Design review of the part built by this model. Coordinates are the model's own, in mm. A direction names the side the tool comes from. Coordinates: 2 decimals unless noted, no trailing zeros. Write each loop counter-clockwise with the first axis right and the second up, starting at its lowest first coordinate (ties: lowest second). Pieces come first, ordered by that corner, then holes. Notation, with made-up numbers: (39.25, 51.25) -> (62.25, 51.25) arc R22 ccw to (62.25, 73.25) -> close; hole circle Ø8 at (-38.5, 70.25). An arc over 180 degrees is marked (long way). One line per question, with ' | ' between items. Start each with the question number.
Q1. Add section C-C on y = 0. State the section outline as (x, z) points, and give its area (3 significant figures).
Q2. For P1, Ø16, axis at x = 17, z = 609, coming from the -Y side; P2, Ø10, axis at x = 46.5, z = 456.5, coming from the +Y side; P3, Ø6, axis at x = 11, y = -98, coming from the -Z side; P4, Ø24, axis at x = 0, z = 730, coming from the +Y side, all flat-tipped, find the tip position at first contact; note any pin that passes through.
Q3. Wall thickness on probe 1 along Z at (x, y) = (0, 104); probe 2 along Y at (x, z) = (-16.5, 681.5); probe 3 along Z at (x, y) = (44, 4): over which ranges is each line inside the solid? List them lowest first.
Q4. For faces 1 (the flat face through (-35, -105, 629)), 2 (the flat face through (35, -105, 629)), 3 (the flat face through (0, 110, 555)), 4 (the flat face through (0, 90, 610)), list the 3-axis set-ups (+Z, -Z, +X, -X, +Y, -Y) from which the entire face can be reached by the end or side of a thin tool; tool diameter is ignored.
Q5. Add section B-B on x = 0. Give the number of separate pieces and of enclosed holes in the cut face, and give its area (3 significant figures).
Q6. Add section A-A on z = 730. State the section outline as (x, y) points, and give its area (3 significant figures).
Q7. Draft analysis for pull direction Y (two halves, no side actions). For faces 5 (the flat face through (0, 120, 692)), 6 (the flat face through (0, 100, 500)), 7 (the flat face through (0, -100, 697)), state which applies: pulls with the +Y half, pulls with the -Y half, needs draft (parallel to the pull), parting line crosses it, or undercut.
Q8. Add section D-D on z = 566.5. State the section outline as (x, y) points.
Autodesk Inventor part; units mm, degrees
ref_plane "YZ Plane" through (0, 0, 0) normal (1, 0, 0) x (0, 1, 0)
ref_plane "XZ Plane" through (0, 0, 0) normal (0, 1, 0) x (-1, 0, 0)
ref_plane "XY Plane" through (0, 0, 0) normal (0, 0, 1) x (1, 0, 0)
sketch "Náčrt1" plane through (0, 0, 0) normal (0, 0, 1) x (1, 0, 0)
  line L0 (-90, -90) -> (90, -90)
  line L1 (90, -90) -> (90, 90)
  line L2 (90, 90) -> (-90, 90)
  line L3 (-90, 90) -> (-90, -90)
  line L4 (-90, -90) -> (90, 90) construction
  line L5 (90, -90) -> (-90, 90) construction
  point P0 (0, 0)
  dimension "d0" = 180
extrude "Vysunutí1" add sketch "Náčrt1" along normal blind 600
sketch "Náčrt2" plane through (0, 0, 0) normal (1, 0, 0) x (0, 1, 0)
  line L0 (-90, 0) -> (-90, 600)
  line L1 (-100, 630) -> (-100, 765)
  line L2 (-120, 681.7157) -> (-120, 540)
  line L3 (-90, 600) -> (90, 600)
  line L4 (0, 600) -> (0, 773.8359) construction
  line L5 (-90, 0) -> (90, 0)
  line L6 (-90, 500) -> (-90, 620)
  line L7 (-90, 620) -> (-100, 630)
  line L8 (-120, 765) -> (-120, 621.7157)
  line L9 (-120, 621.7157) -> (-110, 611.7157)
  line L10 (-110, 611.7157) -> (-110, 500)
  line L11 (-120, 765) -> (-100, 765)
  line L12 (-110, 500) -> (-90, 500)
  line L13 (-120, 730) -> (-100, 730) construction
  point P0 (0, 0)
  dimension "d5" = 100
  dimension "d22" = 135
  dimension "d24" = 20
  dimension "d26" = 20
  dimension "d35" = 35
  dimension "d36" = 130
  dimension "d37" = 100
extrude "Vysunutí2" add sketch "Náčrt2" along normal mid plane 70
sketch "Náčrt3" plane through (-30, -120, 582.0978) normal (0, -1, 0) x (1, 0, 0)
  line L0 (-5, 182.9022) -> (65, 182.9022)
  line L1 (30, 182.9022) -> (30, 119.5637) construction
  circle A0 centre (30, 147.9022) radius 20
  point P0 (30, -582.0978)
  dimension "d11" = 40
  dimension "d12" = 35
  dimension "d25" = 70
extrude "Vysunutí3" cut sketch "Náčrt3" against normal blind 60
chamfer "Zkosení1" distance 10 angle 45 2 edges at (35, -110, 765) (-35, -110, 765)
mirror "Zrcadlit1" about plane through (0, 0, 0) normal (0, 1, 0)
sketch "Náčrt5" plane through (0, 0, 0) normal (0, 0, -1) x (-1, 0, 0)
  circle A0 centre (0, 0) radius 65
  dimension "d40" = 130
extrude "Vysunutí5" add sketch "Náčrt5" along normal blind 20
equation "\"d12\" = 0.5 * d25"
properties part number "B6-A2"
Output values:
1) outline: (-90, 0) -> (-65, 0) -> (-65, -20) -> (65, -20) -> (65, 0) -> (90, 0) -> (90, 600) -> (-90, 600) -> close | area: 111,000 mm2
2) P1: stops at y = -115.28 | P2: stops at y = 90 | P3: stops at z = 500 | P4: passes through
3) probe 1: z = 500 to 710, 750 to 765 | probe 2: y = -120 to -100, 100 to 120 | probe 3: z = -20 to 600
4) face 1: +Z, -Z, -X, -Y | face 2: +Z, -Z, +X, -Y | face 3: -Z, +X, -X, +Y | face 4: +Z, +X, -X
5) separate pieces: 3 | enclosed holes: 0 | area: 120,000 mm2
6) outline: (-35, -120) -> (-20, -120) -> (-20, -100) -> (-35, -100) -> close; (-35, 100) -> (-20, 100) -> (-20, 120) -> (-35, 120) -> close; (20, -120) -> (35, -120) -> (35, -100) -> (20, -100) -> close; (20, 100) -> (35, 100) -> (35, 120) -> (20, 120) -> close | area: 1,200 mm2
7) face 5: pulls with the +Y half | face 6: needs draft | face 7: undercut
8) outline: (-90, -90) -> (-35, -90) -> (-35, -110) -> (35, -110) -> (35, -90) -> (90, -90) -> (90, 90) -> (35, 90) -> (35, 110) -> (-35, 110) -> (-35, 90) -> (-90, 90) -> close
